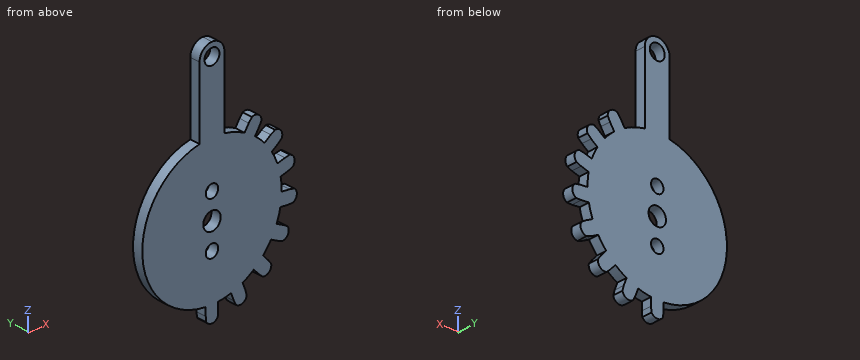
```python
from build123d import *

# Parameters (mm, degrees)
BOSS_EXTRUDE1_DEPTH = 1
SKETCH5_R           = 1.75
SKETCH5_R_2         = 1.25
CUT_EXTRUDE3_DEPTH  = 35.568104475
FILLET1_R           = 2.5
SKETCH6_R           = 1.5
CUT_EXTRUDE4_DEPTH  = 35.568104475


with BuildPart() as part:
    # Sketch1 → Boss-Extrude1 (new, symmetric)
    with BuildSketch(Plane(origin=(0, 0, 0), x_dir=(1, 0, 0), z_dir=(0, 1, 0))):
        with BuildLine():
            Line((1.25, 15.5), (1.15, 16.5))
            ThreePointArc((1.15, 16.5), (0, 17.143895929), (-1.15, 16.5))
            Line((-1.15, 16.5), (-1.25, 15.5))
            Line((-1.25, 15.5), (-1.25, 13.944084767))
            ThreePointArc((-1.25, 13.944084767), (-13.985786559, 0.630693533), (-2.5, -13.774977314))
            Line((-2.5, -13.774977314), (-2.5, -30))
            Line((-2.5, -30), (2.5, -30))
            Line((2.5, -30), (2.5, -13.774977314))
            ThreePointArc((2.5, -13.774977314), (4.576899397, -13.230721519), (6.546154662, -12.375292285))
            Line((6.546154662, -12.375292285), (7.393566833, -13.680192597))
            Line((7.393566833, -13.680192597), (8.022072925, -14.464399261))
            ThreePointArc((8.022072925, -14.464399261), (9.337234935, -14.378080935), (9.951015231, -13.211729481))
            Line((9.951015231, -13.211729481), (9.490243253, -12.318595009))
            Line((9.490243253, -12.318595009), (8.642831082, -11.013694698))
            ThreePointArc((8.642831082, -11.013694698), (9.63696406, -10.155241194), (10.546269982, -9.207398626))
            Line((10.546269982, -9.207398626), (11.805031847, -10.121942654))
            Line((11.805031847, -10.121942654), (12.672827367, -10.628826206))
            ThreePointArc((12.672827367, -10.628826206), (13.869703156, -10.076929194), (14.024733447, -8.768087119))
            Line((14.024733447, -8.768087119), (13.274494978, -8.099400168))
            Line((13.274494978, -8.099400168), (12.015733113, -7.18485614))
            ThreePointArc((12.015733113, -7.18485614), (12.636193981, -6.027155355), (13.145427794, -4.816401987))
            Line((13.145427794, -4.816401987), (14.648326501, -5.219102482))
            Line((14.648326501, -5.219102482), (15.640134232, -5.381328944))
            ThreePointArc((15.640134232, -5.381328944), (16.559731841, -4.437166774), (16.235418036, -3.159699544))
            Line((16.235418036, -3.159699544), (15.295374114, -2.804287916))
            Line((15.295374114, -2.804287916), (13.792475407, -2.401587421))
            ThreePointArc((13.792475407, -2.401587421), (13.956842672, -1.09842734), (13.998358191, 0.214401383))
            Line((13.998358191, 0.214401383), (15.545749957, 0.377038811))
            Line((15.545749957, 0.377038811), (16.529819006, 0.581019464))
            ThreePointArc((16.529819006, 0.581019464), (17.049979873, 1.792025096), (16.289403541, 2.868419824))
            Line((16.289403541, 2.868419824), (15.284428799, 2.86334355))
            Line((15.284428799, 2.86334355), (13.737037033, 2.700706122))
            ThreePointArc((13.737037033, 2.700706122), (13.423476288, 3.976214826), (12.991758626, 5.216723857))
            Line((12.991758626, 5.216723857), (14.37808925, 5.923094591))
            Line((14.37808925, 5.923094591), (15.223696724, 6.466185743))
            ThreePointArc((15.223696724, 6.466185743), (15.275323122, 7.78316588), (14.179518574, 8.515500749))
            Line((14.179518574, 8.515500749), (13.243113, 8.150610901))
            Line((13.243113, 8.150610901), (11.856782377, 7.444240167))
            ThreePointArc((11.856782377, 7.444240167), (11.106946764, 8.522660006), (10.259344927, 9.526061183))
            Line((10.259344927, 9.526061183), (11.30045543, 10.682331537))
            Line((11.30045543, 10.682331537), (11.895271554, 11.492389423))
            ThreePointArc((11.895271554, 11.492389423), (11.471505478, 12.740397548), (10.186038456, 13.031389818))
            Line((10.186038456, 13.031389818), (9.442593367, 12.355158053))
            Line((9.442593367, 12.355158053), (8.401482864, 11.198887699))
            ThreePointArc((8.401482864, 11.198887699), (7.314979906, 11.936962301), (6.164088599, 12.569964667))
            Line((6.164088599, 12.569964667), (6.721678751, 14.022536674))
            Line((6.721678751, 14.022536674), (6.986688658, 14.991953895))
            ThreePointArc((6.986688658, 14.991953895), (6.143822831, 16.005205673), (4.839453677, 15.816200179))
            Line((4.839453677, 15.816200179), (4.387727685, 14.918456548))
            Line((4.387727685, 14.918456548), (3.830137533, 13.465884541))
            ThreePointArc((3.830137533, 13.465884541), (2.551297357, 13.765568706), (1.25, 13.944084767))
            Line((1.25, 13.944084767), (1.25, 15.5))
        make_face()
    extrude(amount=BOSS_EXTRUDE1_DEPTH, both=True)

    # Sketch5 → Cut-Extrude3 (cut, through all)
    with BuildSketch(Plane(origin=(0, 1, 0), x_dir=(1, 0, 0), z_dir=(0, 1, 0))):
        with Locations(Location((0, 0, 0), (0, 0, 270))):
            Circle(SKETCH5_R)
        with Locations(Location((0, 5.011164895, 0), (0, 0, 270))):
            Circle(SKETCH5_R_2)
        with Locations(Location((0, -5.011164895, 0), (0, 0, 90))):
            Circle(SKETCH5_R_2)
    extrude(amount=-CUT_EXTRUDE3_DEPTH, mode=Mode.SUBTRACT)

    # Fillet1
    fillet1_edges = [part.edges().sort_by_distance(p)[0] for p in [
        (-2.5, 0, 30),
        (2.5, 0, 30),
    ]]
    fillet(fillet1_edges, radius=FILLET1_R - 0.0001)  # a hair under: the kernel refuses the full size

    # Sketch6 → Cut-Extrude4 (cut, through all)
    with BuildSketch(Plane(origin=(0, 1, 0), x_dir=(1, 0, 0), z_dir=(0, 1, 0))):
        with Locations(Location((0, -27.5, 0), (0, 0, 270))):
            Circle(SKETCH6_R)
    extrude(amount=-CUT_EXTRUDE4_DEPTH, mode=Mode.SUBTRACT)


solid = part.part
```
For this review, take the finished solid that the model builds, in its own axes (mm). Round coordinates to 2 decimals unless told otherwise and drop trailing zeros. Write each loop counter-clockwise with the first axis right and the second up, starting at its lowest first coordinate (ties: lowest second). Pieces come first, ordered by that corner, then holes. Notation, with made-up numbers: (38, 30) - (65, 30) arc R22 cw to (65, 63) - close; hole circle Ø7 at (58, 80.5). An arc over 180 degrees is marked (long way). Answer as CSV lines item,"result". Start each with the question number.
(1) Add section A-A, the plane z = 1. State the section outline as (x, y) points, plus the area to 3 significant figures.
(2) For line 1 (X direction, y = -0.3, z = 0); line 2 (X direction, y = -0.5, z = 27.5); line 3 (X direction, y = 0.7, z = 17), list the stretches that pass through material, from the lowest coordinate up.
(3) Add section B-B, the plane y = 0.35. State how many separate pieces and enclosed holes the cut face has, plus the area to 3 significant figures.
(4) Add section D-D, the plane x = -8. State the section outline as (y, z) points, plus the area to 3 significant figures.
(5) Add section C-C, the plane z = 23.5. State the section outline as (x, y) points.
(6) For pin 1 (3 mm diameter, centred on x = 0, z = 5.01, fed in from -Y); pin 2 (1 mm diameter, centred on y = -0.5, z = 21.5, fed in from +X); pin 3 (0.5 mm diameter, centred on y = 0.5, z = -14.5, fed in from -X); pin 4 (1 mm diameter, centred on y = -0.5, z = 20.5, fed in from -X), all flat-tipped, find the tip position at first contact; note any pin that passes through.
From the geometry:
1,outline,"(-13.96, -1) - (-1.44, -1) - (-1.44, 1) - (-13.96, 1) - close; (1.44, -1) - (13.96, -1) - (13.96, 1) - (1.44, 1) - close"
1,area,"50.1 mm²"
2,line 1,"x = -14 to -1.75, 1.75 to 14"
2,line 2,"x = -2.5 to -1.5, 1.5 to 2.5"
2,line 3,"x = -2.5 to 2.5"
3,separate pieces,"1"
3,enclosed holes,"4"
3,area,"725 mm²"
4,outline,"(-1, -11.49) - (1, -11.49) - (1, 11.49) - (-1, 11.49) - close"
4,area,"46.0 mm²"
5,outline,"(-2.5, -1) - (2.5, -1) - (2.5, 1) - (-2.5, 1) - close"
6,pin 1,"stops at y = -1"
6,pin 2,"stops at x = 2.5"
6,pin 3,"stops at x = -1.25"
6,pin 4,"stops at x = -2.5"
